Autodesk Inventor part; units mm, degrees
ref_plane "YZ Plane" through (0, 0, 0) normal (1, 0, 0) x (0, 1, 0)
ref_plane "XZ Plane" through (0, 0, 0) normal (0, 1, 0) x (-1, 0, 0)
ref_plane "XY Plane" through (0, 0, 0) normal (0, 0, 1) x (1, 0, 0)
sketch "Náčrt1" plane through (0, 0, 0) normal (0, 1, 0) x (-1, 0, 0)
  line L0 (14, -2) -> (10.9978, 1.0022)
  line L1 (10.9978, 1.0022) -> (-10.9978, 1.0022)
  line L2 (-10.9978, 1.0022) -> (-14, -2)
  line L3 (-14, -2) -> (-26, -2)
  line L4 (-26, -2) -> (-26, 2)
  line L5 (-26, 2) -> (26, 2)
  line L6 (26, 2) -> (26, -2)
  line L7 (26, -2) -> (14, -2)
  line L8 (20, 1.0022) -> (22.6, -0.4989)
  line L9 (22.6, -0.4989) -> (22.6, -3.5011)
  line L10 (22.6, -3.5011) -> (20, -5.0022)
  line L11 (20, -5.0022) -> (17.4, -3.5011)
  line L12 (17.4, -3.5011) -> (17.4, -0.4989)
  line L13 (17.4, -0.4989) -> (20, 1.0022)
  line L14 (-20, 1.0022) -> (-17.4, -0.4989)
  line L15 (-17.4, -0.4989) -> (-17.4, -3.5011)
  line L16 (-17.4, -3.5011) -> (-20, -5.0022)
  line L17 (-20, -5.0022) -> (-22.6, -3.5011)
  line L18 (-22.6, -3.5011) -> (-22.6, -0.4989)
  line L19 (-22.6, -0.4989) -> (-20, 1.0022)
  line L20 (26, 2) -> (0, 0) construction
  line L21 (0, 0) -> (-26, 2) construction
  line L22 (26, -2) -> (0, 0) construction
  line L23 (-17.4, -3.5011) -> (-15.5011, -3.5011)
  line L24 (-15.5011, -3.5011) -> (-14, -2)
  line L25 (17.4, -3.5011) -> (15.5011, -3.5011)
  line L26 (15.5011, -3.5011) -> (14, -2)
  line L27 (-22.6, -3.5011) -> (-24.4989, -3.5011)
  line L28 (-24.4989, -3.5011) -> (-26, -2)
  line L29 (22.6, -3.5011) -> (24.4989, -3.5011)
  line L30 (24.4989, -3.5011) -> (26, -2)
  line L31 (-13, -1) -> (13, -1)
  line L32 (-22.6, -0.4989) -> (-22.6, -0.2989)
  line L33 (-22.6, -0.2989) -> (-20, 1.2022)
  line L34 (-20, 1.2022) -> (-17.4, -0.2989)
  line L35 (-17.4, -0.2989) -> (-17.4, -0.4989)
  line L36 (17.4, -0.4989) -> (17.4, -0.2989)
  line L37 (17.4, -0.2989) -> (20, 1.2022)
  line L38 (20, 1.2022) -> (22.6, -0.2989)
  line L39 (22.6, -0.2989) -> (22.6, -0.4989)
  point P0 (20, -2)
  point P1 (-20, -2)
  dimension "d0" = 5.2
  dimension "d1" = 40
  dimension "d4" = 4
  dimension "d6" = 45
  dimension "d7" = 1
  dimension "d8" = 52
  dimension "d19" = 0.2
  dimension "d20" = 0.2
extrude "Vysunutí1" add sketch "Náčrt1" along normal blind 2.7 contours L0 L1 L2 L3 L15 L35 L34 L33 L32 L18 L4 L5 L6 L7 L9 L39 L38 L37 L36 L12 | L7 L12 L25 L26 | L31 L2 L1 L0 | L7 L30 L29 L9 | L24 L23 L15 L3 | L18 L27 L28 L3
sketch "Náčrt2" plane through (0, 2.7, 0) normal (0, 1, 0) x (1, 0, 0)
  line L0 (-13, 1) -> (-15.5011, 3.5011)
  line L1 (-15.5011, 3.5011) -> (-17.4, 3.5011)
  line L2 (-17.4, 3.5011) -> (-17.4, 0.2989)
  line L3 (-22.6, 0.2989) -> (-22.6, 3.5011)
  line L4 (-22.6, 3.5011) -> (-24.4989, 3.5011)
  line L5 (-24.4989, 3.5011) -> (-26, 2)
  line L6 (-26, 2) -> (-26, -2)
  line L7 (-26, -2) -> (26, -2)
  line L8 (26, -2) -> (26, 2)
  line L9 (26, 2) -> (24.4989, 3.5011)
  line L10 (24.4989, 3.5011) -> (22.6, 3.5011)
  line L11 (22.6, 3.5011) -> (22.6, 0.2989)
  line L12 (17.4, 0.2989) -> (17.4, 3.5011)
  line L13 (17.4, 3.5011) -> (15.5011, 3.5011)
  line L14 (15.5011, 3.5011) -> (13, 1)
  line L15 (13, 1) -> (-13, 1)
  circle A0 centre (-20.075, 1.9567) radius 1.65
  circle A1 centre (20, 2) radius 1.65
  line L16 (-22.75, 0.4123) -> (-20.075, 1.9567) construction
  line L17 (-20.075, 1.9567) -> (-17.4, 0.4123) construction
  line L18 (-20.075, 1.9567) -> (-20.075, -1.1321) construction
  line L19 (20, 2) -> (22.675, 0.4556) construction
  line L20 (20, -1.0888) -> (20, 2) construction
  line L21 (17.325, 0.4556) -> (20, 2) construction
  line L22 (-22.6, 3.5011) -> (-17.4, 3.5011)
  line L23 (22.6, 3.5011) -> (17.4, 3.5011)
  line L24 (18.35, 2) -> (18.35, 3.5011)
  line L25 (21.65, 2) -> (21.65, 3.5011)
  line L26 (-18.425, 1.9567) -> (-18.425, 3.5011)
  line L27 (-21.725, 1.9567) -> (-21.725, 3.5011)
  line L28 (-17.4, 0.2989) -> (-20, -1.2022)
  line L29 (-20, -1.2022) -> (-22.6, 0.2989)
  line L30 (22.6, 0.2989) -> (20, -1.2022)
  line L31 (20, -1.2022) -> (17.4, 0.2989)
  point P0 (0, 0)
  point P1 (19.315, 3.5011)
  point P2 (20.685, 3.5011)
  point P3 (-20.6558, 3.5011)
  point P4 (-19.4942, 3.5011)
  dimension "d11" = 3.3
extrude "Vysunutí2" add sketch "Náčrt2" against normal blind 0.4 contours L2 L28 L29 L3 L22 L27 A0 L26 | L23 L24 A1 L25 L11 L30 L31 L12
sketch "Náčrt3" plane through (13, 0, -1) normal (0, 0, -1) x (-1, 0, 0)
  line L0 (0, 0) -> (26, 0)
  line L1 (26, 0) -> (26, 2.7)
  line L2 (0, 2.7) -> (26, 2.7)
  line L3 (0, 0) -> (0, 2.7)
  line L4 (0, 2.7) -> (1.2124, 2)
  line L5 (1.2124, 2) -> (24.7876, 2)
  line L6 (24.7876, 2) -> (26, 2.7)
  point P0 (13, 0)
  dimension "d14" = 2
  dimension "d16" = 60
extrude "Vysunutí3" cut sketch "Náčrt3" against normal through all contours L2 L6 L5 L4
properties part number "miniboard nutt holder"
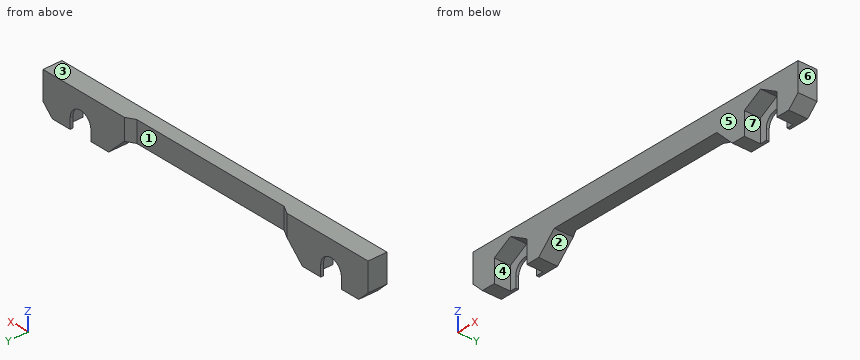
Source: CAD feature listing. Evaluate the final solid. Frame: model axes, mm. Face numbers are marked on the shaded views. A direction names the side the tool comes from. Give positions to 0.01 mm unless a question says otherwise; leave off trailing zeros. Write each loop counter-clockwise with the first axis right and the second up, starting at its lowest first coordinate (ties: lowest second). Pieces come first, ordered by that corner, then holes.
1. Section query A-A (z = -1.45). Return the cut outline in (x, y), then the cut area to 3 significant figures.
2. Access query for the marked faces 1, 2, 3 and 4. Directions: +Z, -Z, +X, -X, +Y, -Y. A direction counts if a zero-diameter tool reaches every point of the face in a straight line with its end or side. Return the directions, or none.
3. First-contact query: pin 1 (2.5 mm diameter, centred on x = -20.5, z = -1, fed in from -Y); pin 2 (1.4 mm diameter, centred on x = -5.5, y = 1.5, fed in from -Z). Flat tips, straight axial feed; report the tip coordinate or a pass-through.
4. Section query D-D (x = -20.5). Return the cut outline in (y, z).
5. Section query C-C (x = 2.5). Return the cut outline in (y, z), then the cut area to 3 significant figures.
6. Material intervals for line 1 along X through (y, z) = (0.5, -0.6); line 2 along X through (y, z) = (2.4, -1.6); line 3 along X through (y, z) = (0.8, -2.3), sorted ascending.
7. Pull-direction query (X, two-part tool) for the marked faces 5, 6 and 7; classes: +X half, -X half, draft (parallel to the pull), parting line (faces both ways), or undercut.
8. Section query B-B (y = 1.55). Return the cut outline in (x, z).
Output values:
1. outline: (-26, 0) - (-22.6, 0) - (-22.6, 2.3) - (-21.65, 2.3) - (-21.65, 2.7) - (-26, 2.7) - close; (-18.5, 2.3) - (-17.4, 2.3) - (-17.4, 0) - (-13.45, 0) - (-13.45, 2.7) - (-18.5, 2.7) - close; (13.45, 0) - (17.4, 0) - (17.4, 2.3) - (18.44, 2.3) - (18.44, 2.7) - (13.45, 2.7) - close; (21.56, 2.3) - (22.6, 2.3) - (22.6, 0) - (26, 0) - (26, 2.7) - (21.56, 2.7) - close
1. area: 41.3 mm2
2. face 1: +Z, -Z, +Y
2. face 2: -Z, +Y, -Y
2. face 3: +Z, +X, -X, +Y, -Y
2. face 4: -Z, -Y
3. pin 1: stops at y = 2.3
3. pin 2: stops at z = -1
4. outline: (0, 0.91) - (2.3, 0.91) - (2.3, -0.36) - (2.7, -0.36) - (2.7, 2) - (0, 2) - close
5. outline: (0, -1) - (2, -1) - (2, 2) - (0, 2) - close
5. area: 6.00 mm2
6. line 1: x = -26 to -22.6, -17.4 to 17.4, 22.6 to 26
6. line 2: x = -26 to -21.69, -18.46 to -13.6, 13.6 to 18.4, 21.6 to 26
6. line 3: x = -25.7 to -22.6, -17.4 to -14.3, 14.3 to 17.4, 22.6 to 25.7
7. face 5: draft
7. face 6: +X half
7. face 7: undercut
8. outline: (-26, -2) - (-24.5, -3.5) - (-22.6, -3.5) - (-22.6, -0.3) - (-20, 1.2) - (-17.4, -0.3) - (-17.4, -3.5) - (-15.5, -3.5) - (-13, -1) - (13, -1) - (15.5, -3.5) - (17.4, -3.5) - (17.4, -0.3) - (20, 1.2) - (22.6, -0.3) - (22.6, -3.5) - (24.5, -3.5) - (26, -2) - (26, 2) - (-26, 2) - close
